from build123d import *

# Parameters (mm, degrees)
CROQUIS1_R              = 2.3
SALIENTE_EXTRUIR1_DEPTH = 7.5
CROQUIS4_R              = 3.925
SALIENTE_EXTRUIR3_DEPTH = 32.5
CROQUIS5_R              = 3.925


with BuildPart() as part:
    # Croquis1 → Saliente-Extruir1 (new body)
    with BuildSketch(Plane.XY):
        with BuildLine():
            Line((3.627068375, 1.5), (7.475, 1.5))
            Line((7.475, 1.5), (7.475, -1.5))
            Line((7.475, -1.5), (3.627068375, -1.5))
            ThreePointArc((3.627068375, -1.5), (0, -3.925), (-3.627068375, -1.5))
            Line((-3.627068375, -1.5), (-7.475, -1.5))
            Line((-7.475, -1.5), (-7.475, 1.5))
            Line((-7.475, 1.5), (-3.627068375, 1.5))
            ThreePointArc((-3.627068375, 1.5), (0, 3.925), (3.627068375, 1.5))
        make_face()
        Circle(CROQUIS1_R, mode=Mode.SUBTRACT)
    extrude(amount=-SALIENTE_EXTRUIR1_DEPTH)

    # Croquis4 → Saliente-Extruir3 (add)
    with BuildSketch(Plane(origin=(0, 0, -7.5), x_dir=(-1, 0, 0), z_dir=(0, 0, -1))):
        with Locations(Location((0, 0, 0), (0, 0, 202.467889888))):
            Circle(CROQUIS4_R)
    extrude(amount=SALIENTE_EXTRUIR3_DEPTH)

    # Barrer2: sweep along a path in Croquis6
    with BuildLine(Plane(origin=(0, 0, 0), x_dir=(1, 0, 0), z_dir=(0, 1, 0))) as barrer2_path:
        Line((0, 40), (23.664319132, 40))
        ThreePointArc((23.664319132, 40), (28.246894827, 42.127016654), (29.580398915, 47))
        ThreePointArc((29.580398915, 47), (0, 72), (-29.580398915, 47))
        ThreePointArc((-29.580398915, 47), (-28.246894827, 42.127016654), (-23.664319132, 40))
        Line((-23.664319132, 40), (0, 40))
    # Croquis5 → Barrer2 (sweep)
    with BuildSketch(Plane(origin=(0, 0, 0), x_dir=(0, 0, -1), z_dir=(1, 0, 0))):
        with Locations((40, 0)):
            Circle(CROQUIS5_R)
    sweep(path=barrer2_path.line)


solid = part.part
The listing builds one solid part. Answer for the finished solid, in the listing's coordinates (mm). A direction names the side the tool comes from. Coordinates: 2 decimals unless noted, no trailing zeros. Order: outer loops, then holes, each group sorted by start corner. A loop starts at its lowest first (then second) coordinate and runs counter-clockwise, first axis right, second up. Notation, with made-up numbers: (9.5, 87.5) -> (34.5, 87.5) arc R11 cw to (34.5, 101.5) -> close; hole circle Ø7 at (10, 82). An arc over 180 degrees is marked (long way). Answer in a Markdown table with one row per item. Add a question column.
Item 1: Find the intervals of material crossed by L1, parallel to Z at x = 6, y = 0.5; L2, parallel to Y at x = 3.5, z = -72; L3, parallel to Y at x = 0, z = -5 (3 decimals), in increasing order. Write a range as from..to.
Item 2: Find section C-C (z = -22). Write down the section's boundary in (x, y) (3 decimals).
Item 3: Which of the six approach directions +Z, -Z, +X, -X, +Y, -Y give full straight-line access (tool end or side, diameter ignored) to faces 4 (the face through (-7.475, 0, -4)), 5 (the face through (6, 1.5, -4)), 6 (the face through (7.475, 0, -4)), 7 (the face through (0.331, 1.179, -43.744))?
Item 4: Each of these flat-tipped pins is pushed along its axis until it touches: P1, Ø1.9, axis at x = 5, z = -2, coming from the +Y side; P2, Ø4, axis at y = 0.5, z = -53, coming from the +X side; P3, Ø1.5, axis at x = 3.5, z = -68, coming from the -Y side. Where does it stop, or does it pass through?
Item 5: Determine the mould class of faces 1 (the face through (-6, 1.5, -4)), 2 (the face through (-6, 0, -7.5)), 3 (the face through (2, -2, 0)) for opening direction Z: +Z half, -Z half, draft (parallel to the pull), parting line (faces both ways), or undercut.
Item 6: Find section A-A (x = 0). Write down the section's boundary in (y, z) (3 decimals).
Result set:
| question | item | result |
|---|---|---|
| 1 | L1 | z = -75.36..-67.41, -43.89..-36.11, -7.5..0 |
| 1 | L2 | y = -3.92..3.92 |
| 1 | L3 | y = -3.925..-2.3, 2.3..3.925 |
| 2 | outline | circle Ø7.85 at (0, 0) |
| 3 | face 4 | +Z, -X, +Y, -Y |
| 3 | face 5 | +Z, +X, +Y |
| 3 | face 6 | +Z, +X, +Y, -Y |
| 3 | face 7 | none |
| 4 | P1 | stops at y = 1.5 |
| 4 | P2 | stops at x = 32.7 |
| 4 | P3 | stops at y = -2.51 |
| 5 | face 1 | draft |
| 5 | face 2 | undercut |
| 5 | face 3 | +Z half |
| 6 | outline | circle Ø7.85 at (0, -72); (-3.925, -40) arc R3.925 ccw to (3.925, -40) -> (3.925, 0) -> (2.3, 0) -> (2.3, -7.5) -> (-2.3, -7.5) -> (-2.3, 0) -> (-3.925, 0) -> close |
